Input: dimensioned drawing with shaded views. Units: mm. Origin: part minimum x, y, z. Round coordinates to 2 decimals unless told otherwise and drop trailing zeros. Write each loop counter-clockwise with the first axis right and the second up, starting at its lowest first coordinate (ties: lowest second). Pieces come first, ordered by that corner, then holes. Notation, with made-up numbers: (26, 30.25) -> (75, 30.25) arc R12 cw to (75, 41.25) -> close; hole circle Ø10 at (-7.75, 79). An arc over 180 degrees is marked (long way). Use one line per item in the form item = value. Start each with the question number.
1. Cut plane B-B, the plane z = 1.4. Return the cut outline in (x, y), plus the area to 3 significant figures.
2. Pin query (flat end, axial travel): pin 1 Ø2.5 at (x, z) = (13, 2.5) entering from +Y; pin 2 Ø3 at (x, z) = (37, 1) entering from -Y; pin 3 Ø2.5 at (y, z) = (72.5, 2.5) entering from +X; pin 4 Ø2.5 at (y, z) = (66, 3) entering from -X. Return the tip coordinate at first contact, or that it passes through.
3. Cut plane A-A, the plane y = 70. Return the cut outline in (x, z).
4. Cut plane D-D, the plane x = 33.5. Return the cut outline in (y, z).
5. Cut plane C-C, the plane y = 33.5. Return the cut outline in (x, z).
6. Line query: L1, parallel to Y at x = 45.5, z = 3.7; L2, parallel to Y at x = 73.5, z = 1.9; L3, parallel to X at y = 69, z = 3.3. Output: solid intervals per line, ascending.
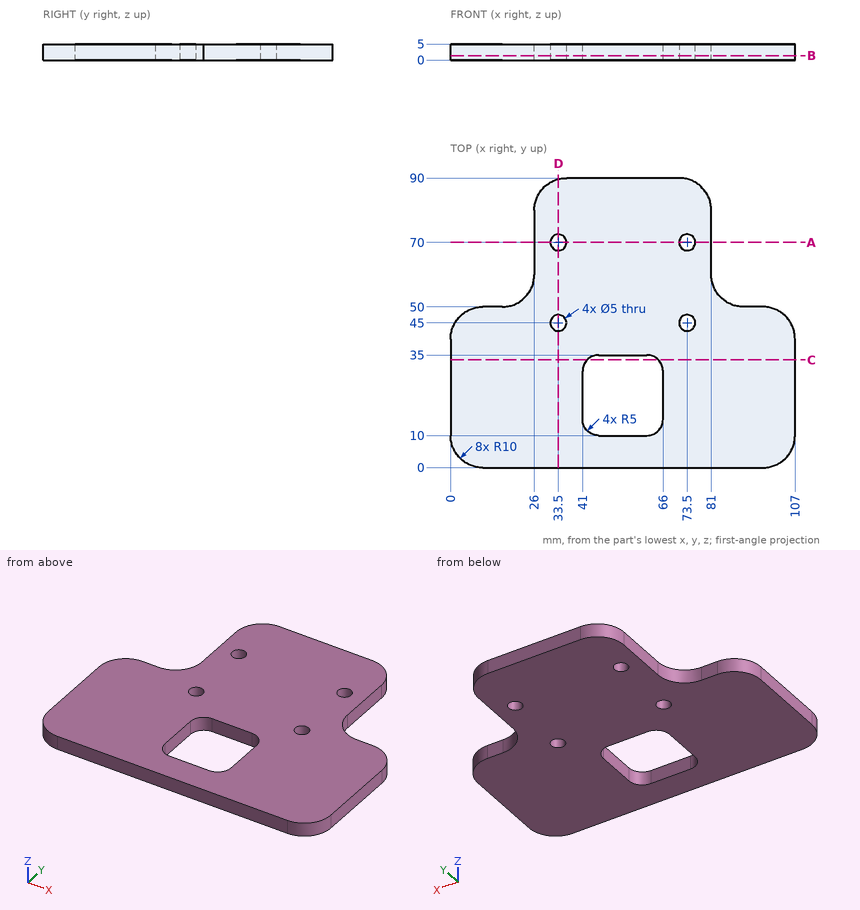
Outcome:
q1.outline = (0, 10) arc R10 ccw to (10, 0) -> (97, 0) arc R10 ccw to (107, 10) -> (107, 40) arc R10 ccw to (97, 50) -> (91, 50) arc R10 cw to (81, 60) -> (81, 80) arc R10 ccw to (71, 90) -> (36, 90) arc R10 ccw to (26, 80) -> (26, 60) arc R10 cw to (16, 50) -> (10, 50) arc R10 ccw to (0, 40) -> close; hole circle Ø5 at (33.5, 45); hole circle Ø5 at (33.5, 70); hole (41, 15) arc R5 ccw to (46, 10) -> (61, 10) arc R5 ccw to (66, 15) -> (66, 30) arc R5 ccw to (61, 35) -> (46, 35) arc R5 ccw to (41, 30) -> close; hole circle Ø5 at (73.5, 45); hole circle Ø5 at (73.5, 70)
q1.area = 6,780 mm^2
q2.pin_1 = 50
q2.pin_2 = 0
q2.pin_3 = 81
q2.pin_4 = 26
q3.outline = (26, 0) -> (31, 0) -> (31, 5) -> (26, 5) -> close; (36, 0) -> (71, 0) -> (71, 5) -> (36, 5) -> close; (76, 0) -> (81, 0) -> (81, 5) -> (76, 5) -> close
q4.outline = (0, 0) -> (42.5, 0) -> (42.5, 5) -> (0, 5) -> close; (47.5, 0) -> (67.5, 0) -> (67.5, 5) -> (47.5, 5) -> close; (72.5, 0) -> (89.68, 0) -> (89.68, 5) -> (72.5, 5) -> close
q5.outline = (0, 0) -> (42.43, 0) -> (42.43, 5) -> (0, 5) -> close; (64.57, 0) -> (107, 0) -> (107, 5) -> (64.57, 5) -> close
q6.L1 = 0 to 10.03, 34.97 to 90
q6.L2 = 0 to 42.5, 47.5 to 67.5, 72.5 to 89.68
q6.L3 = 26 to 31.21, 35.79 to 71.21, 75.79 to 81
